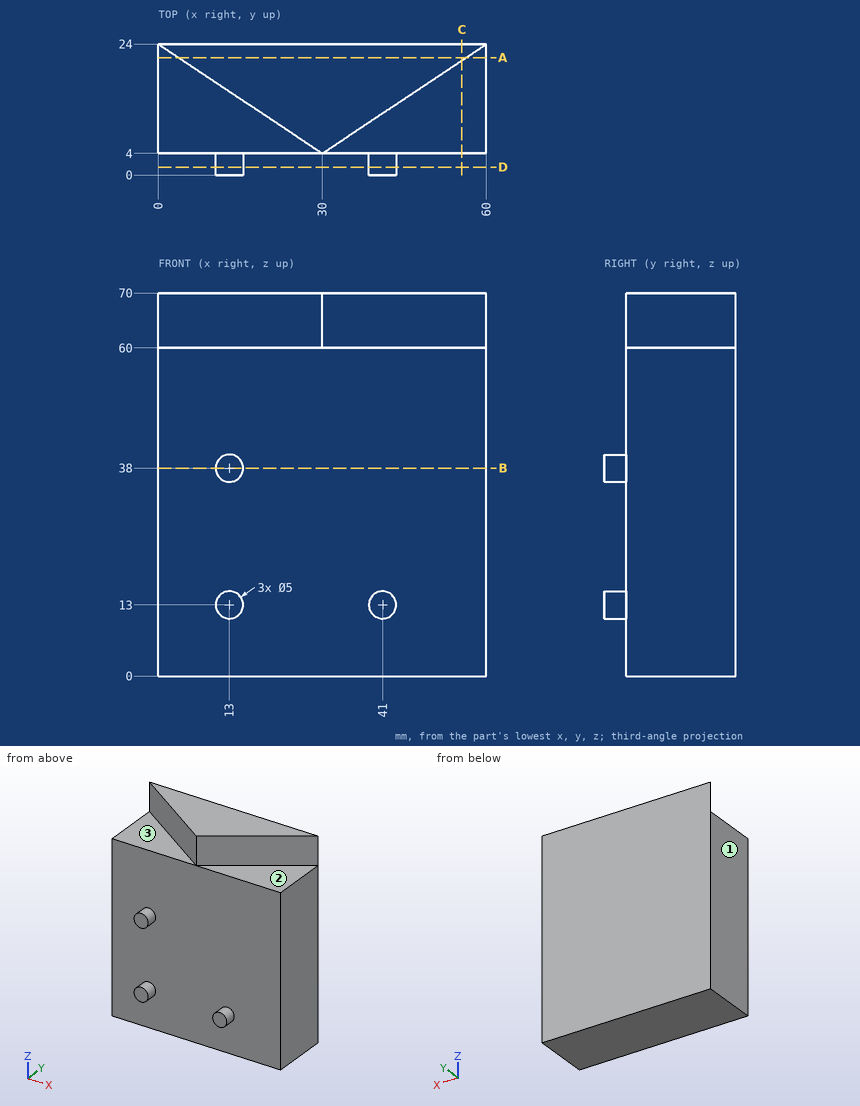
Here's the drawing with two shaded views (mm, measured from the low corner). I have some questions. A direction names the side the tool comes from. Coordinates: 2 decimals unless noted, no trailing zeros. Loops run counter-clockwise (first coordinate to the right, second up) from the corner with the lowest first, then second, coordinate; pieces in that order, holes last. Notation, with made-up numbers: (-22.5, -14) -> (16.5, -14) arc R25 ccw to (16.5, 16) -> close; hole circle Ø2 at (24.25, -23.75). An arc over 180 degrees is marked (long way). Answer in a Markdown table with one row per item.
(1) Imagine slicing it at B-B (z = 38). List the corners of the cut face in (x, y) for me.
Results found:
| item | result |
|---|---|
| outline | (0, 4) -> (10.5, 4) -> (10.5, 0) -> (15.5, 0) -> (15.5, 4) -> (60, 4) -> (60, 24) -> (0, 24) -> close |
(2) For the marked faces 1, 2 and 3, which set-ups out of +Z, -Z, +X, -X, +Y, -Y let a thin tool reach every point of the face, with its end or its side?
Results found:
| item | result |
|---|---|
| face 1 | +Z, -Z, -X, +Y, -Y |
| face 2 | +Z, +X, -Y |
| face 3 | +Z, -X, -Y |
(3) Imagine slicing it at D-D (y = 1.5). List the corners of the cut face in (x, z) for me.
Results found:
| item | result |
|---|---|
| outline | circle Ø5 at (13, 13); circle Ø5 at (13, 38); circle Ø5 at (41, 13) |
(4) Imagine slicing it at A-A (y = 21.5). List the corners of the cut face in (x, z) for me.
Results found:
| item | result |
|---|---|
| outline | (0, 0) -> (60, 0) -> (60, 60) -> (56.25, 60) -> (56.25, 70) -> (3.75, 70) -> (3.75, 60) -> (0, 60) -> close |
(5) Will these pins go through, and if not, where does the flat tip stop? pin 1 Ø8 at (x, z) = (46.5, 57.5) entering from -Y; pin 2 Ø3 at (x, y) = (48.5, 5) entering from +Z.
Results found:
| item | result |
|---|---|
| pin 1 | stops at y = 4 |
| pin 2 | stops at z = 60 |
(6) Imagine slicing it at C-C (x = 55.5). List the corners of the cut face in (y, z) for me, plus the area to 3 significant figures.
Results found:
| item | result |
|---|---|
| outline | (4, 0) -> (24, 0) -> (24, 70) -> (21, 70) -> (21, 60) -> (4, 60) -> close |
| area | 1,230 mm^2 |
(7) If I drill on probe 1 along Z at (x, y) = (18, 4.75); probe 2 along Y at (x, z) = (57, 7.5); probe 3 along Y at (x, z) = (7, 67.5), over which ranges is the centre line in solid material (lowest first)?
Results found:
| item | result |
|---|---|
| probe 1 | z = 0 to 60 |
| probe 2 | y = 4 to 24 |
| probe 3 | y = 19.33 to 24 |
